The figure shows three views and two pictorial views of one solid part (mm, origin at its lowest corner). Answer the questions. Give positions to 0.01 mm unless a question says otherwise; leave off trailing zeros. Write each loop counter-clockwise with the first axis right and the second up, starting at its lowest first coordinate (ties: lowest second). Pieces come first, ordered by that corner, then holes. Notation, with made-up numbers: (-40, 48) -> (7, 48) arc R27 cw to (7, 85) -> close; hole circle Ø8 at (-24.5, 80). An arc over 180 degrees is marked (long way). Use a Markdown table: item, result.
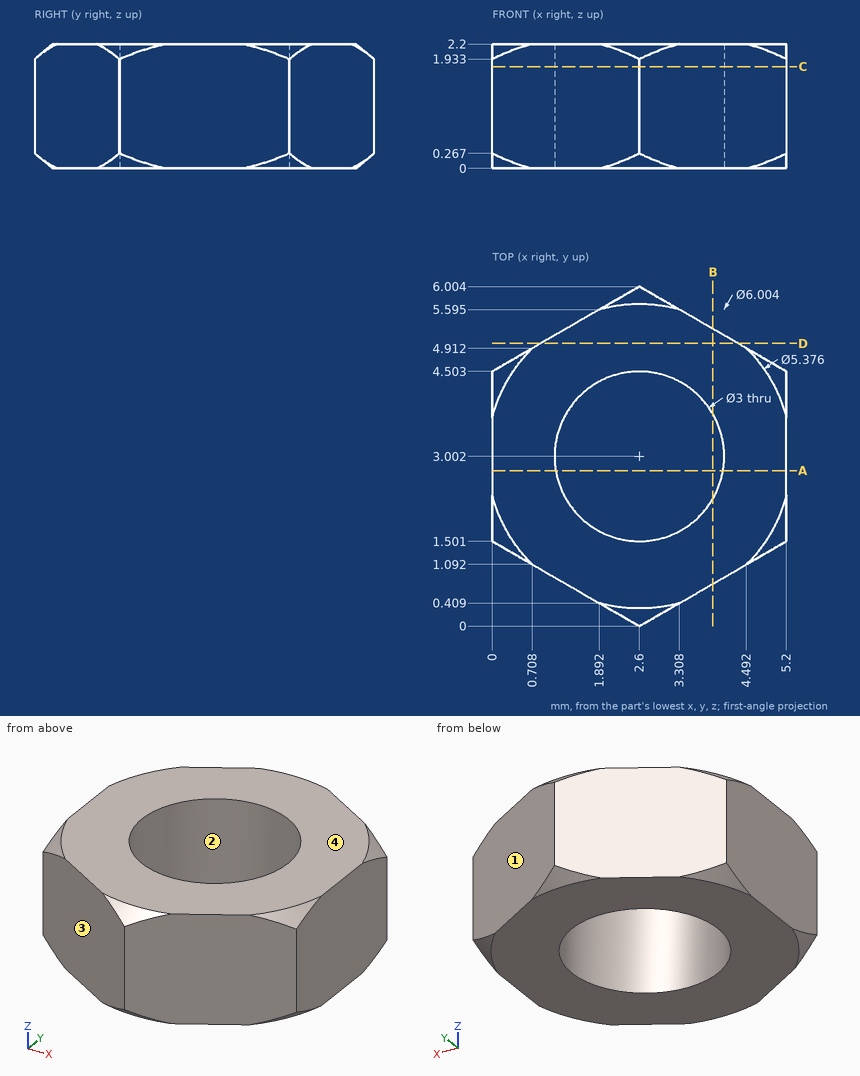
Item 1: For a pull along Y with two mould halves and no side action, classify the marked faces 1, 2, 3 and 4 as +Y half, -Y half, draft (parallel to the pull), parting line (faces both ways), or undercut.
Return value:
| item | result |
|---|---|
| face 1 | +Y half |
| face 2 | undercut |
| face 3 | -Y half |
| face 4 | draft |
Item 2: A cutting plane is placed at A-A (y = 2.75). Give the vertices of the cut face in (x, z).
Return value:
| item | result |
|---|---|
| outline | (0, 0) -> (1.12, 0) -> (1.12, 2.2) -> (0, 2.2) -> close; (4.08, 0) -> (5.2, 0) -> (5.2, 2.2) -> (4.08, 2.2) -> close |
Item 3: A cutting plane is placed at D-D (y = 5). Give the vertices of the cut face in (x, z).
Return value:
| item | result |
|---|---|
| outline | (0.86, 0) -> (4.34, 0) -> (4.34, 2.2) -> (0.86, 2.2) -> close |
Item 4: A cutting plane is placed at B-B (x = 3.9). Give the vertices of the cut face in (y, z).
Return value:
| item | result |
|---|---|
| outline | (0.75, 0) -> (2.25, 0) -> (2.25, 2.2) -> (0.75, 2.2) -> close; (3.75, 0) -> (5.25, 0) -> (5.25, 2.2) -> (3.75, 2.2) -> close |
Item 5: Straight lines are drawn through the part: line 1 along X through (y, z) = (3, 0.45); line 2 along X through (y, z) = (3.75, 1.65); line 3 along Y through (x, z) = (3, 0.9) (1 decimal). For each, find the intervals that lie inside material, in ascending order. Write a range as [from, to].
Return value:
| item | result |
|---|---|
| line 1 | [0, 1.1], [4.1, 5.2] |
| line 2 | [0, 1.3], [3.9, 5.2] |
| line 3 | [0.2, 1.6], [4.4, 5.8] |
Item 6: A cutting plane is placed at C-C (z = 1.8). Give the vertices of the cut face in (x, y) (1 decimal).
Return value:
| item | result |
|---|---|
| outline | (0, 1.5) -> (2.6, 0) -> (5.2, 1.5) -> (5.2, 4.5) -> (2.6, 6) -> (0, 4.5) -> close; hole circle Ø3 at (2.6, 3) |
